Autodesk Inventor part; units mm, degrees
ref_plane "YZ Plane" through (0, 0, 0) normal (1, 0, 0) x (0, 1, 0)
ref_plane "XZ Plane" through (0, 0, 0) normal (0, 1, 0) x (-1, 0, 0)
ref_plane "XY Plane" through (0, 0, 0) normal (0, 0, 1) x (1, 0, 0)
sketch "Sketch1" plane through (0, 0, 0) normal (0, 1, 0) x (-1, 0, 0)
  line L0 (0, 0) -> (-64.77, 0)
  line L1 (-64.77, 0) -> (-64.77, -57.15)
  line L2 (-64.77, -57.15) -> (0, -57.15)
  line L3 (0, -57.15) -> (0, 0)
  dimension "d0" = 64.77
  dimension "d1" = 57.15
extrude "Extrusion1" add sketch "Sketch1" along normal blind 34.9368
sketch "Sketch2" plane through (0, 34.9368, 0) normal (0, 1, 0) x (1, 0, 0)
  circle A0 centre (33.2953, 13.7711) radius 1.27
  line L0 (0, 0) -> (64.77, 0)
  line L1 (0, 57.15) -> (0, 0)
  circle A1 centre (18.8349, 28.2314) radius 1.27
  circle A2 centre (36.3358, 45.7323) radius 1.27
  line L2 (64.77, 57.15) -> (0, 57.15)
  circle A3 centre (50.7961, 31.2719) radius 1.27
  dimension "d4" = 13.7711
  dimension "d5" = 33.2953
  dimension "d6" = 2.54
  dimension "d7" = 2.54
  dimension "d8" = 28.2314
  dimension "d9" = 18.8349
  dimension "d10" = 2.54
  dimension "d11" = 11.4177
  dimension "d12" = 36.3358
  dimension "d13" = 2.54
  dimension "d14" = 25.8781
  dimension "d15" = 50.7961
hole "Hole1" at (50.7961, 34.9368, -31.2719) at (36.3358, 34.9368, -45.7323) at (18.8349, 34.9368, -28.2314) at (33.2953, 34.9368, -13.7711) direction (0, -1, 0) diameter 1.567 end through all
sketch "Sketch3" plane through (0, 34.9368, 0) normal (0, 1, 0) x (1, 0, 0)
  circle A0 centre (6.8509, 12.5984) radius 1.27
  line L0 (0, 0) -> (64.77, 0)
  line L1 (0, 57.15) -> (0, 0)
  circle A1 centre (6.8509, 37.9984) radius 1.27
  circle A2 centre (57.6509, 37.9984) radius 1.27
  circle A3 centre (57.6509, 12.5984) radius 1.27
  dimension "d23" = 2.54
  dimension "d24" = 12.5984
  dimension "d25" = 6.8509
  dimension "d26" = 2.54
  dimension "d27" = 25.4
  dimension "d28" = 2.54
  dimension "d29" = 50.8
  dimension "d30" = 2.54
  dimension "d31" = 50.8
hole "Hole2" at (57.6509, 34.9368, -37.9984) at (57.6509, 34.9368, -12.5984) at (6.8509, 34.9368, -12.5984) at (6.8509, 34.9368, -37.9984) direction (0, -1, 0) diameter 6.7564 end through all counterbore diameter 11.1252 counterbore depth 6.35
sketch "Sketch4" plane through (0, 34.9368, 0) normal (0, 1, 0) x (1, 0, 0)
  line L0 (15.7866, 37.911) -> (27.2166, 49.341)
  line L1 (27.2166, 49.341) -> (24.6766, 51.881)
  line L2 (24.6766, 51.881) -> (13.2466, 40.451)
  line L3 (13.2466, 40.451) -> (15.7866, 37.911)
  line L4 (0, 57.15) -> (0, 0)
  dimension "d39" = 45
  dimension "d40" = 24.7669
  dimension "d41" = 2.54
  dimension "d42" = 11.43
extrude "Extrusion2" add sketch "Sketch4" along normal blind 3.81
sketch "Sketch5" plane through (0, 34.9368, 0) normal (0, 1, 0) x (1, 0, 0)
  line L0 (47.9873, 39.0305) -> (35.2873, 51.7305)
  line L1 (35.2873, 51.7305) -> (37.8273, 54.2705)
  line L2 (37.8273, 54.2705) -> (50.5273, 41.5705)
  line L3 (50.5273, 41.5705) -> (47.9873, 39.0305)
  line L4 (64.77, 0) -> (64.77, 57.15)
  point P0 (0, 0)
  dimension "d45" = 2.54
  dimension "d46" = 12.7
  dimension "d47" = 45
  dimension "d48" = 24.6795
extrude "Extrusion3" add sketch "Sketch5" along normal blind 3.81
properties part number "ResGalvoMount_base_plate"
Check sheet for the modelled part. Datum: model origin and axes. Units: mm. A direction names the side the tool comes from. Round coordinates to 2 decimals unless told otherwise and drop trailing zeros. Order: outer loops, then holes, each group sorted by start corner. A loop starts at its lowest first (then second) coordinate and runs counter-clockwise, first axis right, second up. Notation, with made-up numbers: (-18.75, 27) - (5.25, 27) arc R24 cw to (5.25, 50) - close; hole circle Ø6 at (-30, 14.25). An arc over 180 degrees is marked (long way). Answer as CSV lines item,"result". Start each with the question number.
1) Section check C-C (y = 3). Give the number of separate pieces and of enclosed holes in the cut face, then the cut area to 3 significant figures.
2) Section check D-D (z = -48). Record the cut outline in (x, y).
3) Scan lines: probe 1 along X at (y, z) = (9, -38); probe 2 along Z at (x, y) = (60.5, 12); probe 3 along Z at (x, y) = (58.5, 32). Record each from-to range of solid material in increasing order.
4) Depth check by flat-ended pin: pin 1 (1 mm diameter, centred on y = 23.5, z = -34.5, fed in from -X); pin 2 (12 mm diameter, centred on x = 7, z = -10.5, fed in from +Y); pin 3 (10 mm diameter, centred on x = 6.85, z = -38, fed in from +Y); pin 4 (1.3 mm diameter, centred on x = 50.8, z = -31.27, fed in from -Y). Enter the tip coordinate at first touch or a pass-through.
5) Draft check along X on faces 1 (the face through (0, 17, -29)), 2 (the face through (20, 38.747, -45)), 3 (the face through (10.5, 28.587, -12.7)), 4 (the face through (32.52, 17.22, -13.87)). Enter one of: +X half, -X half, draft (parallel to the pull), parting line (faces both ways), or undercut.
6) Section check A-A (y = 36). Record the cut outline in (x, z), then the cut area to 3 significant figures.
7) Section check B-B (x = 60). Record the cut outline in (y, z), then the cut area to 3 significant figures.
8) Tool access check on faces 5 (the face through (19.042, 36.815, -46.246)), 6 (the face through (58, 28.587, -34)), 7 (the face through (25.964, 36.815, -50.593)), 8 (the face through (41.73, 36.82, -45.29)). Record the directions out of +Z, -Z, +X, -X, +Y, -Y that give a thin tool (end or side, any length) a straight path to the whole face; none if there is none.
Determined:
1,separate pieces,"1"
1,enclosed holes,"8"
1,area,"3,550 mm^2"
2,outline,"(0, 0) - (64.77, 0) - (64.77, 34.94) - (44.1, 34.94) - (44.1, 38.75) - (39.02, 38.75) - (39.02, 34.94) - (25.88, 34.94) - (25.88, 38.75) - (20.8, 38.75) - (20.8, 34.94) - (0, 34.94) - close"
3,probe 1,"0 to 3.47, 10.23 to 54.27, 61.03 to 64.77"
3,probe 2,"-57.15 to -39.81, -36.18 to -14.41, -10.78 to 0"
3,probe 3,"-57.15 to -43.5, -32.5 to -18.1, -7.1 to 0"
4,pin 1,"x = 0"
4,pin 2,"y = 34.94"
4,pin 3,"y = 28.59"
4,pin 4,"through"
5,face 1,"-X half"
5,face 2,"draft"
5,face 3,"undercut"
5,face 4,"undercut"
6,outline,"(13.25, -40.45) - (24.68, -51.88) - (27.22, -49.34) - (15.79, -37.91) - close; (35.29, -51.73) - (37.83, -54.27) - (50.53, -41.57) - (47.99, -39.03) - close"
6,area,"123 mm^2"
7,outline,"(0, -57.15) - (34.94, -57.15) - (34.94, -43.04) - (28.59, -43.04) - (28.59, -40.43) - (0, -40.43) - close; (0, -35.57) - (28.59, -35.57) - (28.59, -32.96) - (34.94, -32.96) - (34.94, -17.64) - (28.59, -17.64) - (28.59, -15.03) - (0, -15.03) - close; (0, -10.17) - (28.59, -10.17) - (28.59, -7.56) - (34.94, -7.56) - (34.94, 0) - (0, 0) - close"
7,area,"1,590 mm^2"
8,face 5,"-Z, -X, +Y"
8,face 6,"+Y"
8,face 7,"-Z, +Y"
8,face 8,"+Z, +Y"
